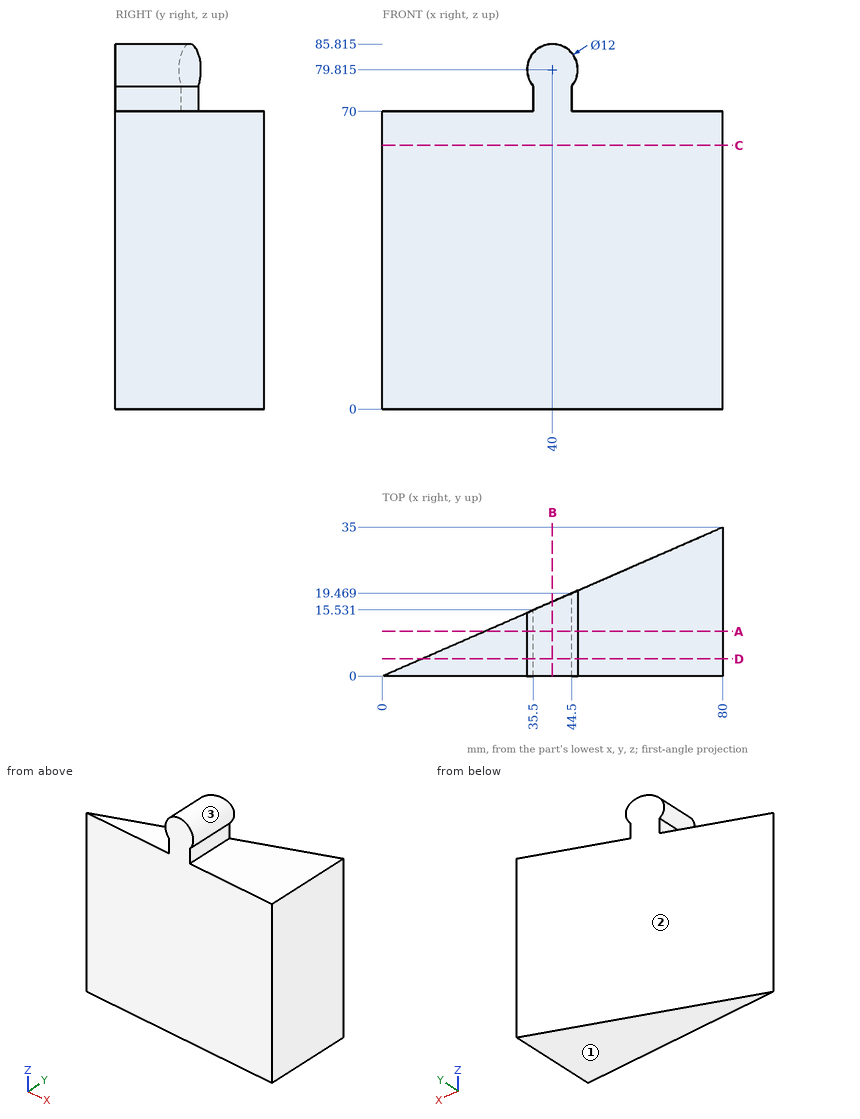
Could you check a few things on this drawing? It's one solid part, dimensions in mm from its lowest x, y, z. Round coordinates to 2 decimals unless told otherwise and drop trailing zeros. Write each loop counter-clockwise with the first axis right and the second up, starting at its lowest first coordinate (ties: lowest second). Pieces come first, ordered by that corner, then holes.
Q1. If we section it at B-B on x = 40: Write out the boundary of the cut face in (y, z) (1 decimal), plus the area to 3 significant figures.
Q2. If we section it at C-C on z = 62: Write out the boundary of the cut face in (x, y).
Q3. Will these pins go through, and if not, where does the flat tip stop? P1, Ø10, axis at x = 51.5, z = 13, coming from the +Y side; P2, Ø1.8, axis at y = 5.5, z = 73.5, coming from the +X side; P3, Ø17.5, axis at x = 70.5, y = 23.5, coming from the +Z side.
Q4. If we section it at A-A on y = 10.5: Write out the boundary of the cut face in (x, z) (1 decimal), plus the area to 3 significant figures.
Q5. Please list where these lines run through material, in increasing order: probe 1 along Z at (x, y) = (73.5, 2); probe 2 along X at (y, z) = (3, 57.5) (1 decimal); probe 3 along X at (y, z) = (33, 34).
Q6. If we section it at D-D on y = 4: Write out the boundary of the cut face in (x, z) (1 decimal), plus the area to 3 significant figures.
Q7. If we mould it in two halves opening along Z, with no side actions, what happens to the marked faces 1, 2 and 3? For each: +Z half, -Z half, draft (parallel to the pull), parting line (faces both ways), or undercut.
Answer below:
1. outline: (0, 0) - (17.5, 0) - (17.5, 85.8) - (0, 85.8) - close
1. area: 1,500 mm2
2. outline: (0, 0) - (80, 0) - (80, 35) - close
3. P1: stops at y = 24.72
3. P2: stops at x = 44.5
3. P3: stops at z = 70
4. outline: (24, 0) - (80, 0) - (80, 70) - (44.5, 70) - (44.5, 75.8) arc R6 ccw (long way) to (35.5, 75.8) - (35.5, 70) - (24, 70) - close
4. area: 4,070 mm2
5. probe 1: z = 0 to 70
5. probe 2: x = 6.9 to 80
5. probe 3: x = 75.43 to 80
6. outline: (9.1, 0) - (80, 0) - (80, 70) - (44.5, 70) - (44.5, 75.8) arc R6 ccw (long way) to (35.5, 75.8) - (35.5, 70) - (9.1, 70) - close
6. area: 5,110 mm2
7. face 1: -Z half
7. face 2: draft
7. face 3: undercut
